Source: CAD feature listing. Evaluate the final solid. Frame: model axes, mm. A direction names the side the tool comes from. Give positions to 0.01 mm unless a question says otherwise; leave off trailing zeros. Write each loop counter-clockwise with the first axis right and the second up, starting at its lowest first coordinate (ties: lowest second). Pieces come first, ordered by that corner, then holes.
```python
from build123d import *

# Parameters (mm, degrees)
F2_DEPTH = 8.2582915228
F4_COUNT = 5
F5_ANGLE = 30


with BuildPart() as f2:
    # F1 (on Front) → F2 (new body, through all)
    with BuildSketch(Plane.XZ):
        Polygon((0, 10.3923048454), (-6, 0), (6, 0), align=None)
    extrude(amount=F2_DEPTH)

    # F4: F2 ×5 about axis
    f4_axis = Axis((0, 0, 5.1961524227), (0, 0, 1))


with BuildPart() as f2_1:
    add(f2.part)
    for i in range(1, F4_COUNT):
        add(f2.part.rotate(f4_axis, i * 360 / F4_COUNT))


with BuildPart() as f2_2:
    # F5: moved
    add(f2_1.part.rotate(Axis((0, 0, 0), (0, 0, 1)), F5_ANGLE))


solid = f2_2.part
```
1. Section query C-C (y = -5). Return loops of the section in (x, z).
2. Section query A-A (z = 5.5). Return loops of the section in (x, y), plus the area to 3 significant figures.
3. Pull-direction query (X, two-part tool) for faces 5 (the flat face through (4.06, -7.19, 4.11)), 6 (the flat face through (-2.68, -5.53, 7.43)), 7 (the flat face through (-6.09, 0.84, 7.43)); classes: pulls with the +X half, pulls with the -X half, needs draft (parallel to the pull), parting line crosses it, or undercut.
4. Section query D-D (z = 1.5). Return loops of the section in (x, y), plus the area to 3 significant figures.
5. Access query for faces 1 (the flat face through (1.55, -5.93, 7.58)), 2 (the flat face through (4.433, -4.261, 7.433)), 3 (the flat face through (-5.16, -3.302, 7.578)), 4 (the flat face through (-1.082, 6.053, 7.433)). Directions: +Z, -Z, +X, -X, +Y, -Y. A direction counts if a zero-diameter tool reaches every point of the face in a straight line with its end or side. Return the directions, or none.
6. Section query B-B (x = 1.75). Return loops of the section in (y, z).
7. Line query: probe 1 along X at (y, z) = (-8.75, 3); probe 2 along Y at (x, z) = (-9, 1.25); probe 3 along Y at (x, z) = (5, 7.75). Output: solid intervals per line, ascending.
8. Pin query (flat end, axial travel): P1, Ø3, axis at x = 6, z = 5, coming from the -Y side; P2, Ø3, axis at y = 1, z = 5, coming from the -X side; P3, Ø4, axis at y = -7, z = 7, coming from the -X side. Return the tip coordinate at first contact, or that it passes through.
The answers:
1. outline: (-6.79, 0) - (7.86, 0) - (7.86, 2.94) - (2.89, 10.39) - (-0.53, 5.27) - (-4.5, 10.39) - (-6.79, 7.45) - close
2. outline: (-8.69, 0.78) - (-4.7, -1) - (-7.62, -4.25) - (-3.43, -8.03) - (-0.5, -4.78) - (1.68, -8.56) - (6.58, -5.74) - (4.39, -1.95) - (8.67, -1.05) - (7.49, 4.48) - (3.22, 3.57) - (3.67, 7.92) - (-1.95, 8.51) - (-2.4, 4.16) - (-6.4, 5.94) - close
2. area: 178 mm2
3. face 5: pulls with the +X half
3. face 6: undercut
3. face 7: pulls with the -X half
4. outline: (-9.63, -1.33) - (-8.54, -1.82) - (-9.34, -2.7) - (-1.71, -9.57) - (-0.91, -8.69) - (-0.32, -9.72) - (8.58, -4.58) - (7.98, -3.55) - (9.15, -3.3) - (7.01, 6.74) - (5.84, 6.49) - (5.97, 7.68) - (-4.24, 8.75) - (-4.37, 7.56) - (-5.46, 8.05) - close
4. area: 243 mm2
5. face 1: +Z, -Y
5. face 2: +Z, +X
5. face 3: +Z, -X
5. face 4: +Z, +Y
6. outline: (-8.53, 0) - (8.12, 0) - (8.12, 8.85) - (1.94, 7.73) - (0.37, 10.39) - (-0.78, 8.44) - (-3.03, 10.39) - (-8.53, 5.63) - close
7. probe 1: x = -2.62 to -2.14, 0.12 to 1.36
7. probe 2: y = -3.01 to -2.11, -1.77 to 0.09
7. probe 3: y = -6.65 to -5.61, -0.5 to 2.62
8. P1: stops at y = -6.94
8. P2: stops at x = -9.06
8. P3: stops at x = -6.79
